from build123d import *

# Parameters (mm, degrees)
F0_W     = 60.96
F0_H     = 104.14
F0_R     = 17.78
F0_W_2   = 50.8
F0_H_2   = 36.4836389199
F1_DEPTH = 10
F2_R     = 5.07999


# Not quite as in the source:
# - a fillet or chamfer is up to 0.001 mm smaller than in the source, because OpenCascade refuses the exact size


with BuildPart() as f1:
    # F0 (on Front) → F1 (new body)
    with BuildSketch(Plane.XZ):
        Rectangle(F0_W, F0_H)
        with Locations((0, -21.59)):
            Circle(F0_R, mode=Mode.SUBTRACT)
        with Locations((0, 26.67)):
            Rectangle(F0_W_2, F0_H_2, mode=Mode.SUBTRACT)
    extrude(amount=F1_DEPTH)

    # F2 (radius 5.08 in the source; OpenCascade refuses exactly that, so slightly less here)
    f2_edges = [f1.edges().sort_by_distance(p)[0] for p in [
        (-30.48, -5, 52.07),
        (-30.48, -5, -52.07),
        (30.48, -5, 52.07),
        (-30.48, 0, 0),
        (30.48, 0, 0),
        (30.48, -5, -52.07),
    ]]
    fillet(f2_edges, radius=F2_R)


solid = f1.part
Input: part model. Units: mm. Frame: model coordinates. A direction names the side the tool comes from. Coordinates: 2 decimals unless noted, no trailing zeros. Write each loop counter-clockwise with the first axis right and the second up, starting at its lowest first coordinate (ties: lowest second). Pieces come first, ordered by that corner, then holes. Notation, with made-up numbers: M 25.25,-1.75 L 41.25,-1.75 A22 cw 41.25,35.25 Z; hole C -25.75,33 d5. An arc over 180 degrees is marked long. Answer as a JSON object with one key per item and string values. Group by question number.
(1) Section B-B on x = -23.5. Output: boundary loops of the cut face in (y, z).
(2) Ray query, line 1 along Z through (x, y) = (0, -6); line 2 along Z through (x, y) = (-11, -2); line 3 along Z through (x, y) = (-19, -8). Return the intervals inside material, ascending. Write a range as [from, to].
(3) Section D-D on y = -1. Output: boundary loops of the cut face in (x, z).
(4) Set-up query: faces 1 (the face through (25.4, -5, 26)), 2 (the face through (0, -5, -52.07)). Return all of +Z, -Z, +X, -X, +Y, -Y with unobstructed straight access to the full face (end or side cutting, diameter ignored); none if empty.
(5) Contact query for a flat-ended pin moving along its axis: P1, Ø8, axis at x = -18, z = 29.5, coming from the -Y side. Output: stop coordinate, or through.
(6) Mould query, pull axis X, two halves, no side actions, for faces 3 (the face through (30.48, -8, -1)), 4 (the face through (-29.031, -6.181, -50.542)), 5 (the face through (-25.4, -5, 26)). Classes: pulls with the +X half, pulls with the -X half, needs draft (parallel to the pull), parting line crosses it, or undercut.
(7) Section C-C on x = 0. Output: boundary loops of the cut face in (y, z), plus the area to 3 significant figures.
Result set:
{
 "1": {"outline": "M -10,-52.07 L 0,-52.07 L 0,8.43 L -10,8.43 Z; M -10,44.91 L 0,44.91 L 0,52.07 L -10,52.07 Z"},
 "2": {"line 1": "z = [-52.07, -39.37], [-3.81, 8.43], [44.91, 52.07]", "line 2": "z = [-52.07, -35.56], [-7.62, 8.43], [44.91, 52.07]", "line 3": "z = [-52.07, 8.43], [44.91, 52.07]"},
 "3": {"outline": "M -28.43,-51.07 A5.08 ccw -25.4,-52.07 L 25.4,-52.07 A5.08 ccw 28.43,-51.07 L 28.43,51.07 A5.08 ccw 25.4,52.07 L -25.4,52.07 A5.08 ccw -28.43,51.07 Z; hole M -25.4,8.43 L 25.4,8.43 L 25.4,44.91 L -25.4,44.91 Z; hole C 0,-21.59 d35.56"},
 "4": {"face 1": "+Y, -Y", "face 2": "-Z, +X, -X, +Y, -Y"},
 "5": {"P1": "passes through"},
 "6": {"face 3": "pulls with the +X half", "face 4": "pulls with the -X half", "face 5": "undercut"},
 "7": {"outline": "M -10,-52.07 L 0,-52.07 L 0,-39.37 L -10,-39.37 Z; M -10,-3.81 L 0,-3.81 L 0,8.43 L -10,8.43 Z; M -10,44.91 L 0,44.91 L 0,52.07 L -10,52.07 Z", "area": "321 mm2"}
}
